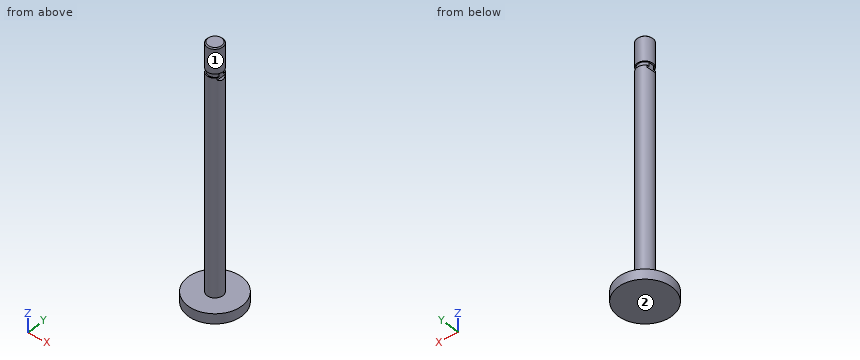
```python
from build123d import *

# Parameters (mm, degrees)
SKETCH1_R        = 3.9624
EXTRUDE1_DEPTH   = 125.2855
SKETCH2_R        = 13.49375
PISTON_DEPTH     = 2.5
FLATS_DEPTH      = 14.49375
FLATS_DEPTH_BACK = 14.49375


with BuildPart() as part:
    # Sketch1 → Extrude1 (new body)
    with BuildSketch(Plane.XY):
        Circle(SKETCH1_R)
    extrude(amount=EXTRUDE1_DEPTH)

    # Sketch2 → Piston (add, symmetric)
    with BuildSketch(Plane.XY):
        Circle(SKETCH2_R)
    extrude(amount=PISTON_DEPTH, both=True)

    # Sketch3 → Threads (revolve, cut)
    with BuildSketch(Plane(origin=(0, 0, 0), x_dir=(0, 0, -1), z_dir=(1, 0, 0))):
        Polygon((-125.2855, 13.49375), (-110.5855, 13.49375), (-110.5855, 3.46), (-112.5855, 3.46), (-112.5855, 3.96), (-124.7855, 3.96), (-125.2855, 3.46), align=None)
    revolve(axis=Axis((0, 0, 0), (0, 0, 1)), mode=Mode.SUBTRACT)

    # Sketch4 → Flats (cut, two sides)
    with BuildSketch(Plane(origin=(0, 0, 0), x_dir=(1, 0, 0), z_dir=(0, 1, 0))) as flats_sk:
        Polygon((3.9624, -112.5855), (3.175, -112.5855), (3.175, -109.5375), (3.9624, -108.7501), align=None)
        Polygon((-3.9624, -108.7501), (-3.9624, -112.5855), (-3.175, -112.5855), (-3.175, -109.5375), align=None)
    extrude(amount=FLATS_DEPTH, mode=Mode.SUBTRACT)
    extrude(flats_sk.sketch, amount=-FLATS_DEPTH_BACK, mode=Mode.SUBTRACT)


solid = part.part
```
Model file for the job. Use its own axes, mm. Face numbers are marked on the shaded views. A direction names the side the tool comes from. Give positions to 0.01 mm unless a question says otherwise; leave off trailing zeros. Order: outer loops, then holes, each group sorted by start corner. A loop starts at its lowest first (then second) coordinate and runs counter-clockwise, first axis right, second up.
1) 3-axis set-ups, long thin cutter, end or side, ignore diameter. For the marked faces 1 and 2: which of +Z, -Z, +X, -X, +Y, -Y reach the whole face in a straight line?
2) Wall check: probe 1 along Z at (x, y) = (-6.5, -1); probe 2 along Y at (x, z) = (-0.25, 88); probe 3 along Z at (x, y) = (-1, -3.75). Give the ranges that are in metal, low to high.
3) Pin check, flat tips, straight feed: pin 1 (12 mm diameter, centred on y = 0.5, z = 23, fed in from -X); pin 2 (1.5 mm diameter, centred on y = 1, z = 110.5, fed in from +X) (3 decimals); pin 3 (8 mm diameter, centred on x = -3, z = 47, fed in from +Y). Stop position of each tip, or through.
4) Saw through at D-D, the plane x = 9.75. Write the cut outline in (y, z).
5) Saw through at A-A, the plane x = 0. Write the cut outline in (y, z), then the cut area to 3 significant figures.
6) Saw through at B-B, the plane y = 0. Write the cut outline in (x, z) (1 decimal), then the cut area to 3 significant figures.
7) Saw through at C-C, the plane z = 29. Write the cut outline in (x, y), then the cut area to 3 significant figures.
Computed:
1. face 1: +Z
1. face 2: -Z, +X, -X, +Y, -Y
2. probe 1: z = -2.5 to 2.5
2. probe 2: y = -3.95 to 3.95
2. probe 3: z = -2.5 to 110.59, 112.59 to 124.86
3. pin 1: stops at x = -3.96
3. pin 2: stops at x = 3.175
3. pin 3: stops at y = 3.96
4. outline: (-9.33, -2.5) - (9.33, -2.5) - (9.33, 2.5) - (-9.33, 2.5) - close
5. outline: (-13.49, -2.5) - (13.49, -2.5) - (13.49, 2.5) - (3.96, 2.5) - (3.96, 110.59) - (3.46, 110.59) - (3.46, 112.59) - (3.96, 112.59) - (3.96, 124.79) - (3.46, 125.29) - (-3.46, 125.29) - (-3.96, 124.79) - (-3.96, 112.59) - (-3.46, 112.59) - (-3.46, 110.59) - (-3.96, 110.59) - (-3.96, 2.5) - (-13.49, 2.5) - close
5. area: 1,110 mm2
6. outline: (-13.5, -2.5) - (13.5, -2.5) - (13.5, 2.5) - (4, 2.5) - (4, 108.8) - (3.2, 109.5) - (3.2, 112.6) - (4, 112.6) - (4, 124.8) - (3.5, 125.3) - (-3.5, 125.3) - (-4, 124.8) - (-4, 112.6) - (-3.2, 112.6) - (-3.2, 109.5) - (-4, 108.8) - (-4, 2.5) - (-13.5, 2.5) - close
6. area: 1,100 mm2
7. outline: circle Ø7.92 at (0, 0)
7. area: 49.3 mm2
